Build history of the part. All positions in model axes, mm. A direction names the side the tool comes from. Give positions to 0.01 mm unless a question says otherwise; leave off trailing zeros. Order: outer loops, then holes, each group sorted by start corner. A loop starts at its lowest first (then second) coordinate and runs counter-clockwise, first axis right, second up. Notation, with made-up numbers: (-24.5, 57) - (30.5, 57) arc R6 ccw to (30.5, 61) - close; hole circle Ø3 at (16.5, -22). An arc over 180 degrees is marked (long way). Use a Markdown table: item, result. Add a question column.
(1) Slice it at B-B (x = -17). Write the cut outline in (y, z), then the cut area to 3 significant figures.
(2) Slice it at D-D (z = 3.3). Count the separate pieces of the cut face and the enclosed holes in it, then the cut area to 3 significant figures.
(3) Mould opens along X. For faces 3 (the face through (-11.925, 2.776, 3.438)), 4 (the face through (-11, 0, 2.794)), 5 (the face through (-25.4, -0.1, 2)), 6 (the face through (25.4, 0.1, 2)) say: +X half, -X half, draft (parallel to the pull), parting line (faces both ways), or undercut.
(4) Slice it at C-C (y = 1.25). Write the cut outline in (x, z) (3 decimals), then the cut area to 3 significant figures.
(5) Slice it at A-A (z = 1.15). Write the cut outline in (x, y).
(6) Flat gauge pin, fed straight in: pin 1 (2 mm diameter, centred on x = -9.5, y = -0.5, fed in from +Z). Where does the tip first touch, or does it go through?
(7) Which spindle directions (+Z, -Z, +X, -X, +Y, -Y) get a long thin tool onto all of the face, cutting with end or side? Do faces 1 (the face through (22.08, -1.26, 1.55)), 2 (the face through (-11.736, -2.763, 3.438)). Say none if no direction does.
(8) Wall check: line 1 (X direction, y = 0, z = 0.9); line 2 (X direction, y = 0, z = 3.3); line 3 (Y direction, x = 19.05, z = 1.5). Give the ranges that are in metal, low to high.
from build123d import *

# Parameters (mm, degrees)
SKETCH1_R           = 3.286877418
SKETCH1_R_2         = 3.282339501
BOSS_EXTRUDE2_DEPTH = 4.064
CUT_EXTRUDE1_DEPTH  = 1.27
CUT_EXTRUDE2_DEPTH  = 5.064


with BuildPart() as part:
    # Sketch1 → Boss-Extrude2 (new body)
    with BuildSketch(Plane.XY):
        with BuildLine():
            Line((-19.05, 6.35), (19.05, 6.35))
            ThreePointArc((19.05, 6.35), (25.4, 0), (19.05, -6.35))
            Line((19.05, -6.35), (-19.05, -6.35))
            ThreePointArc((-19.05, -6.35), (-25.4, 0), (-19.05, 6.35))
        make_face()
        with Locations((-19.05, 0)):
            Circle(SKETCH1_R, mode=Mode.SUBTRACT)
        with Locations((19.05, 0)):
            Circle(SKETCH1_R_2, mode=Mode.SUBTRACT)
    extrude(amount=BOSS_EXTRUDE2_DEPTH)

    # Sketch2 → Cut-Extrude1 (cut)
    with BuildSketch(Plane.XY.offset(4.064)):
        with BuildLine():
            Line((-19.05, 3.286877418), (-5.08, 2.286))
            ThreePointArc((-5.08, 2.286), (-2.794, 0), (-5.08, -2.286))
            Line((-5.08, -2.286), (-19.05, -3.286877418))
            Line((-19.05, -3.286877418), (-19.05, 3.286877418))
        make_face()
        with BuildLine():
            Line((19.05, -3.286877418), (5.08, -2.286))
            ThreePointArc((5.08, -2.286), (2.794, 0), (5.08, 2.286))
            Line((5.08, 2.286), (19.05, 3.286877418))
            Line((19.05, 3.286877418), (19.05, -3.286877418))
        make_face()
    extrude(amount=-CUT_EXTRUDE1_DEPTH, mode=Mode.SUBTRACT)

    # Sketch4 → Cut-Extrude2 (cut, through all)
    with BuildSketch(Plane.XY.offset(4.064)):
        with BuildLine():
            ThreePointArc((18.437330889, 6.35), (73.326339368, 39.20432916), (94.889393238, 99.430942082))
            ThreePointArc((94.889393238, 99.430942082), (-60.226612922, 172.75728145), (-18.437330889, 6.35))
            Line((-18.437330889, 6.35), (18.437330889, 6.35))
        make_face()
        with BuildLine():
            Line((18.437330889, 6.35), (-18.437330889, 6.35))
            ThreePointArc((-18.437330889, 6.35), (-18.146321247, 6.29282972), (-17.855134345, 6.236569254))
            ThreePointArc((-17.855134345, 6.236569254), (-1.97e-07, 4.541548843), (17.855133958, 6.23656918))
            ThreePointArc((17.855133958, 6.23656918), (18.146321054, 6.292829682), (18.437330889, 6.35))
        make_face()
        with BuildLine():
            ThreePointArc((18.437330889, -6.35), (18.146321056, -6.292829683), (17.855133961, -6.236569181))
            ThreePointArc((17.855133961, -6.236569181), (-1.46e-07, -4.541548843), (-17.855134248, -6.236569236))
            ThreePointArc((-17.855134248, -6.236569236), (-18.146321199, -6.292829711), (-18.437330889, -6.35))
            Line((-18.437330889, -6.35), (18.437330889, -6.35))
        make_face()
        with BuildLine():
            Line((18.437330889, -6.35), (-18.437330889, -6.35))
            ThreePointArc((-18.437330889, -6.35), (-60.226612922, -172.75728145), (94.889393238, -99.430942082))
            ThreePointArc((94.889393238, -99.430942082), (73.326339368, -39.20432916), (18.437330889, -6.35))
        make_face()
    extrude(amount=-CUT_EXTRUDE2_DEPTH, mode=Mode.SUBTRACT)


solid = part.part
Solution:
| question | item | result |
|---|---|---|
| 1 | outline | (-6.08, 0) - (-2.57, 0) - (-2.57, 2.79) - (-3.14, 2.79) - (-3.14, 4.06) - (-6.08, 4.06) - close; (2.57, 0) - (6.08, 0) - (6.08, 4.06) - (3.14, 4.06) - (3.14, 2.79) - (2.57, 2.79) - close |
| 1 | area | 27.1 mm2 |
| 2 | separate pieces | 1 |
| 2 | enclosed holes | 2 |
| 2 | area | 315 mm2 |
| 3 | face 3 | undercut |
| 3 | face 4 | undercut |
| 3 | face 5 | -X half |
| 3 | face 6 | +X half |
| 4 | outline | (-25.276, 0) - (-22.09, 0) - (-22.09, 4.064) - (-25.276, 4.064) - close; (-16.01, 0) - (16.015, 0) - (16.015, 2.794) - (3.166, 2.794) - (3.166, 4.064) - (-3.166, 4.064) - (-3.166, 2.794) - (-16.01, 2.794) - close; (22.085, 0) - (25.276, 0) - (25.276, 4.064) - (22.085, 4.064) - close |
| 4 | area | 123 mm2 |
| 5 | outline | (-19.05, -6.35) - (-18.44, -6.35) arc R94.89 cw to (-17.86, -6.24) arc R94.89 cw to (17.86, -6.24) arc R94.89 cw to (18.44, -6.35) - (19.05, -6.35) arc R6.35 ccw to (19.05, 6.35) - (18.44, 6.35) arc R94.89 cw to (17.86, 6.24) arc R94.89 cw to (-17.86, 6.24) arc R94.89 cw to (-18.44, 6.35) - (-19.05, 6.35) arc R6.35 ccw to start; hole circle Ø6.57 at (-19.05, 0); hole circle Ø6.56 at (19.05, 0) |
| 6 | pin 1 | z = 2.79 |
| 7 | face 1 | +Z, -Z |
| 7 | face 2 | +Z |
| 8 | line 1 | -25.4 to -22.34, -15.76 to 15.77, 22.33 to 25.4 |
| 8 | line 2 | -25.4 to -22.34, -2.79 to 2.79, 22.33 to 25.4 |
| 8 | line 3 | -6.35 to -3.28, 3.28 to 6.35 |
